```python
from build123d import *

# Parameters (mm, degrees)
SKETCH2_W               = 7.9
SKETCH2_H               = 1.060956176
CUT_EXTRUDE1_DEPTH      = 4.95
CUT_EXTRUDE1_DEPTH_BACK = 4.95
SKETCH3_R               = 1.5
CUT_EXTRUDE2_DEPTH      = 6.778087647


with BuildPart() as part:
    # Sketch1 → Revolve4 (revolve)
    with BuildSketch(Plane(origin=(0, 0, 0), x_dir=(1, 0, 0), z_dir=(0, 1, 0))):
        with BuildLine():
            Line((0, -3.95), (0, 3.95))
            ThreePointArc((0, 3.95), (3.95, 0), (0, -3.95))
        make_face()
    revolve(axis=Axis((0, 0, 3.95), (0, 0, -1)))

    # Sketch2 → Cut-Extrude1 (cut, two sides)
    with BuildSketch(Plane(origin=(0, 0, 0), x_dir=(1, 0, 0), z_dir=(0, 1, 0))) as cut_extrude1_sk:
        with Locations((0, -3.419521912)):
            Rectangle(SKETCH2_W, SKETCH2_H)
        with Locations((0, 3.419521912)):
            Rectangle(SKETCH2_W, SKETCH2_H)
    extrude(amount=CUT_EXTRUDE1_DEPTH, mode=Mode.SUBTRACT)
    extrude(cut_extrude1_sk.sketch, amount=-CUT_EXTRUDE1_DEPTH_BACK, mode=Mode.SUBTRACT)

    # Sketch3 → Cut-Extrude2 (cut, through all)
    with BuildSketch(Plane.XY.offset(2.889043824)):
        Circle(SKETCH3_R)
    extrude(amount=-CUT_EXTRUDE2_DEPTH, mode=Mode.SUBTRACT)


solid = part.part
```
Verification items for the finished model (mm, model axes). Coordinates: 2 decimals unless noted, no trailing zeros. Loops run counter-clockwise (first coordinate to the right, second up) from the corner with the lowest first, then second, coordinate; pieces in that order, holes last. Notation, with made-up numbers: (-17.5, 16) - (-1.5, 16) arc R29 ccw to (-1.5, 51) - close; hole circle Ø4 at (71.25, -7.75). An arc over 180 degrees is marked (long way). Answer as a JSON object with one key per item and string values.
(1) Cross-section at A-A, the plane x = 0. Record the boundary of the cut face in (y, z), then the cut area to 3 significant figures.
Response:
{"outline": "(-2.69, -2.89) - (-1.5, -2.89) - (-1.5, 2.89) - (-2.69, 2.89) arc R3.95 ccw to start; (1.5, -2.89) - (2.69, -2.89) arc R3.95 ccw to (2.69, 2.89) - (1.5, 2.89) - close", "area": "23.8 mm²"}
(2) Go/stop test with flat-tipped pins: pin 1 Ø1 at (x, z) = (1, -2) entering from +Y; pin 2 Ø2 at (y, z) = (1, -1.5) entering from +X; pin 3 Ø3 at (x, z) = (-2, 0) entering from +Y. Record where each tip stops, or that it passes through.
Response:
{"pin 1": "stops at y = 3.55", "pin 2": "stops at x = 3.87", "pin 3": "stops at y = 3.92"}
(3) Cross-section at C-C, the plane z = -1.05. Record the boundary of the cut face in (x, y).
Response:
{"outline": "circle Ø7.62 at (0, 0); hole circle Ø3 at (0, 0)"}
(4) Mould release check, pull along Y, two halves, no side actions. Record for faces 1 (the flat face through (1.2, -1.2, 2.889)), 2 (the cylindrical face through (-1.5, 0.07, 0.04)): pulls with the +Y half, pulls with the -Y half, needs draft (parallel to the pull), parting line crosses it, or undercut.
Response:
{"face 1": "needs draft", "face 2": "undercut"}
(5) Cross-section at D-D, the plane x = 2.5. Record the boundary of the cut face in (y, z), then the cut area to 3 significant figures.
Response:
{"outline": "(-1, -2.89) - (1, -2.89) arc R3.06 ccw to (1, 2.89) - (-1, 2.89) arc R3.06 ccw to start", "area": "28.9 mm²"}
(6) Scan lines: line 1 along X through (y, z) = (-1.25, -0.45); line 2 along Y through (x, z) = (0, 0.15); line 3 along Y through (x, z) = (0, -1.4). Record each from-to range of solid material in increasing order.
Response:
{"line 1": "x = -3.72 to -0.83, 0.83 to 3.72", "line 2": "y = -3.95 to -1.5, 1.5 to 3.95", "line 3": "y = -3.69 to -1.5, 1.5 to 3.69"}
